Can you work these out from the drawing? Everything is in mm from the part's minimum corner. A direction names the side the tool comes from. Round coordinates to 2 decimals unless told otherwise and drop trailing zeros. Write each loop counter-clockwise with the first axis right and the second up, starting at its lowest first coordinate (ties: lowest second). Pieces come first, ordered by that corner, then holes. Notation, with made-up numbers: M 19,38.25 L 65,38.25 A26 cw 65,74.25 Z; hole C -5.75,33 d2. An arc over 180 degrees is marked long. Answer in a Markdown table with one row per item. Add a question column.
(1) I'm going to push flat-ended pins straight in: pin 1 (12 mm diameter, centred on x = 31.75, z = 14.25, fed in from -Y); pin 2 (3 mm diameter, centred on x = 32, y = 4.5, fed in from +Z); pin 3 (1.5 mm diameter, centred on y = 2, z = 54.5, fed in from -X); pin 4 (1.5 mm diameter, centred on x = 51, y = 3, fed in from +Z). Where does each tip first touch, or does it pass through?
(2) Suppose I cut it at C-C, the plane x = 50. Write out the boundary of the cut face in (y, z).
(3) If we mould it in two halves opening along Z, with no side actions, what happens to the marked faces 3, 4 and 5? For each: released by +Z, released by -Z, zero draft, split by the parting line, or undercut.
(4) Suppose I cut it at B-B, the plane z = 31.75. Write out the boundary of the cut face in (x, y).
(5) Suppose I cut it at D-D, the plane y = 0.8. Count the separate pieces of the cut face and the enclosed holes in it, then the cut area to 3 significant figures.
(6) Suppose I cut it at A-A, the plane x = 31.75. Write out the boundary of the cut face in (y, z).
(7) For the marked faces 1 and 2, which set-ups out of +Z, -Z, +X, -X, +Y, -Y let a thin tool reach every point of the face, with its end or its side?
(8) If I drill on probe 1 along X at (y, z) = (1.3, 19) (1 decimal); probe 2 along X at (y, z) = (0.35, 31.5); probe 3 along X at (y, z) = (4.4, 25) (1 decimal), over which ranges is the centre line in solid material (lowest first)?
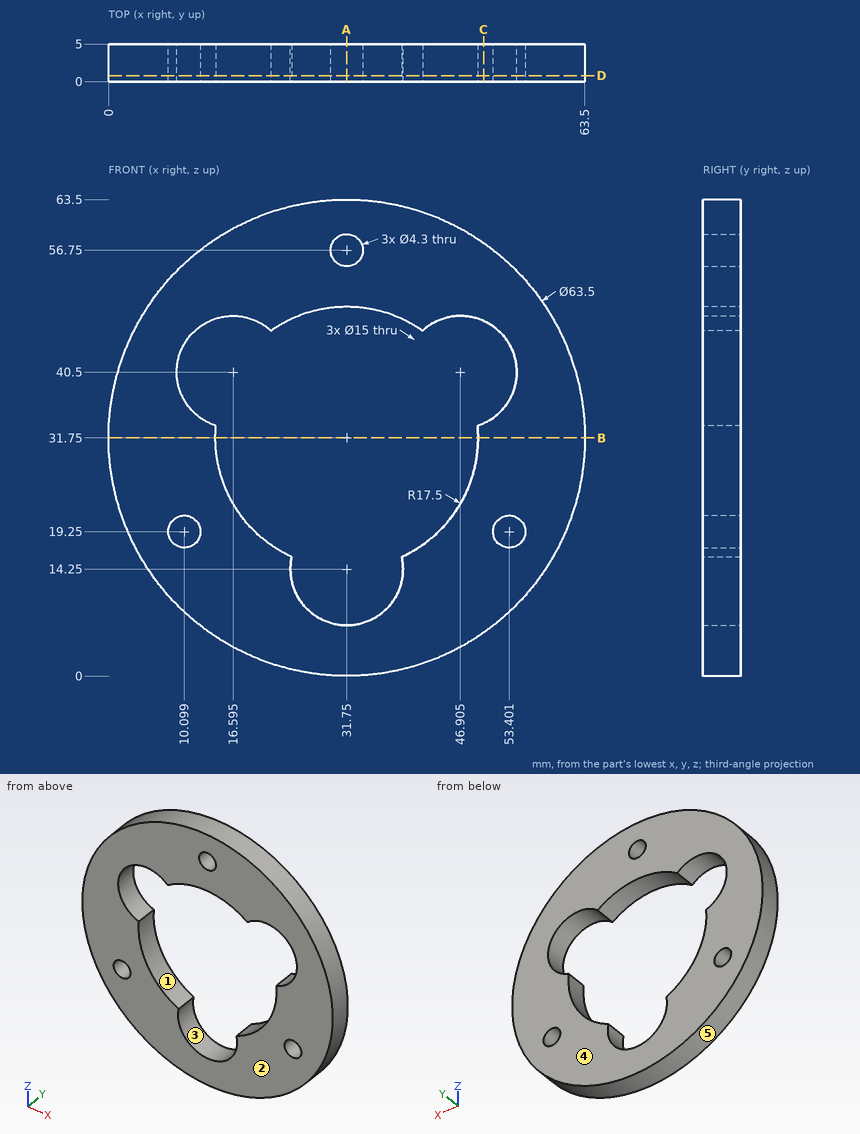
Calculated:
| question | item | result |
|---|---|---|
| 1 | pin 1 | through |
| 1 | pin 2 | z = 63.5 |
| 1 | pin 3 | x = 8.86 |
| 1 | pin 4 | z = 57.55 |
| 2 | outline | M 0,5.77 L 5,5.77 L 5,33.67 L 0,33.67 Z; M 0,47.33 L 5,47.33 L 5,57.73 L 0,57.73 Z |
| 3 | face 3 | undercut |
| 3 | face 4 | zero draft |
| 3 | face 5 | split by the parting line |
| 4 | outline | M 0,0 L 14.25,0 L 14.25,5 L 0,5 Z; M 49.25,0 L 63.5,0 L 63.5,5 L 49.25,5 Z |
| 5 | separate pieces | 1 |
| 5 | enclosed holes | 4 |
| 5 | area | 1,870 mm² |
| 6 | outline | M 0,0 L 5,0 L 5,6.75 L 0,6.75 Z; M 0,49.25 L 5,49.25 L 5,54.6 L 0,54.6 Z; M 0,58.9 L 5,58.9 L 5,63.5 L 0,63.5 Z |
| 7 | face 1 | +Y, -Y |
| 7 | face 2 | +Z, -Z, +X, -X, -Y |
| 8 | probe 1 | 2.7 to 8, 12.2 to 19.8, 43.7 to 51.3, 55.5 to 60.8 |
| 8 | probe 2 | 0 to 14.25, 49.25 to 63.5 |
| 8 | probe 3 | 0.7 to 15.6, 47.9 to 62.8 |
